from build123d import *

# Parameters (mm, degrees)
F1_DEPTH = 20
F3_DEPTH = 20.001
F4_W     = 2.488287
F4_H     = 23.197157
F5_DEPTH = 2.5


with BuildPart() as f1:
    # F0 (on Front) → F1 (new body)
    with BuildSketch(Plane.XZ):
        Polygon((-7.5, -7.5), (7.5, -7.5), (7.5, 7.5), (2, 7.5), (0, 7.5), (-7.5, 7.5), align=None)
    extrude(amount=F1_DEPTH)

    # F2 (on face) → F3 (cut, through all)
    with BuildSketch(Plane(origin=(0, 0, 0), x_dir=(-1, 0, 0), z_dir=(0, 1, 0))):
        with BuildLine():
            Line((-1.379276, 0), (0, 0))
            Line((0, 0), (1.379276, 0))
            ThreePointArc((1.379276, 0), (1.838281, 0.660448), (2, 1.448309))
            ThreePointArc((2, 1.448309), (-0.787861, 3.286589), (-1.379276, 0))
        make_face()
        with BuildLine():
            Line((1.379276, 0), (0, 0))
            Line((0, 0), (-1.379276, 0))
            ThreePointArc((-1.379276, 0), (-1.20038, -0.151406), (-1.005, -0.280846))
            ThreePointArc((-1.005, -0.280846), (0, -0.551691), (1.005, -0.280846))
            ThreePointArc((1.005, -0.280846), (1.20038, -0.151406), (1.379276, 0))
        make_face()
        with BuildLine():
            Line((2.01, 0), (1.379276, 0))
            ThreePointArc((1.379276, 0), (1.20038, -0.151406), (1.005, -0.280846))
            ThreePointArc((1.005, -0.280846), (1.489572, -0.078898), (2.01, -0.01))
            Line((2.01, -0.01), (2.01, 0))
        make_face()
        with BuildLine():
            ThreePointArc((-1.005, -0.280846), (-1.20038, -0.151406), (-1.379276, 0))
            Line((-1.379276, 0), (-2.01, 0))
            Line((-2.01, 0), (-2.01, -0.01))
            ThreePointArc((-2.01, -0.01), (-1.489572, -0.078898), (-1.005, -0.280846))
        make_face()
        with BuildLine():
            ThreePointArc((2.01, -0.01), (1.489572, -0.078898), (1.005, -0.280846))
            ThreePointArc((1.005, -0.280846), (1.012503, -3.743494), (4.01, -2.01))
            ThreePointArc((4.01, -2.01), (3.424214, -0.595786), (2.01, -0.01))
        make_face()
        with BuildLine():
            ThreePointArc((-0.01, -2.01), (-0.276506, -1.012503), (-1.005, -0.280846))
            ThreePointArc((-1.005, -0.280846), (-1.489572, -0.078898), (-2.01, -0.01))
            ThreePointArc((-2.01, -0.01), (-3.424214, -3.424214), (-0.01, -2.01))
        make_face()
    extrude(amount=-F3_DEPTH, mode=Mode.SUBTRACT)

    # F4 (on Top) → F5 (cut)
    with BuildSketch(Plane.XY):
        with Locations((0.051259, -9.1946)):
            Rectangle(F4_W, F4_H)
    extrude(amount=-F5_DEPTH, mode=Mode.SUBTRACT)


solid = f1.part
Geometry check sheet. Reference: the model listing, model coordinates, mm. Round coordinates to 2 decimals unless told otherwise and drop trailing zeros. Write each loop counter-clockwise with the first axis right and the second up, starting at its lowest first coordinate (ties: lowest second). Pieces come first, ordered by that corner, then holes. Notation, with made-up numbers: (-17, 42) - (7, 42) arc R26 cw to (7, 70) - close; hole circle Ø5 at (23.25, 12.25). An arc over 180 degrees is marked (long way). One line per item, written item: value.
1. Cross-section at B-B on z = 2. Record the boundary of the cut face in (x, y).
The answers:
outline: (-7.5, -20) - (-1.92, -20) - (-1.92, 0) - (-7.5, 0) - close; (1.92, -20) - (7.5, -20) - (7.5, 0) - (1.92, 0) - close
2. Cross-section at C-C on z = -0.75. Record the boundary of the cut face in (x, y).
The answers:
outline: (-7.5, -20) - (-3.56, -20) - (-3.56, 0) - (-7.5, 0) - close; (3.56, -20) - (7.5, -20) - (7.5, 0) - (3.56, 0) - close
3. Scan lines: L1, parallel to X at y = -6.25, z = -2.01; L2, parallel to Z at x = 0, y = -11; L3, parallel to X at y = -1.5, z = 1.5. Record each from-to range of solid material in increasing order.
The answers:
L1: x = -7.5 to -4.01, 4.01 to 7.5
L2: z = -7.5 to -2.5, 3.45 to 7.5
L3: x = -7.5 to -2, 2 to 7.5
4. Mould release check, pull along X, two halves, no side actions. Record for faces 1 (the face through (-7.5, -10, 0)), 2 (the face through (0, -10, 7.5)), 3 (the face through (3.626, -9.86, -3.189)): released by +X, released by -X, zero draft, split by the parting line, or undercut.
The answers:
face 1: released by -X
face 2: zero draft
face 3: undercut
5. Depth check by flat-ended pin: pin 1 Ø1.5 at (x, z) = (-1, -4) entering from +Y. Enter the tip coordinate at first touch or a pass-through.
The answers:
pin 1: stops at y = 0
